from build123d import *

# Parameters (mm, degrees)
BOSS_EXTRUDE2_DEPTH      = 10
BOSS_EXTRUDE2_DEPTH_BACK = 14
SKETCH2_R                = 25
SKETCH4_R                = 62.5
BOSS_EXTRUDE3_DEPTH      = 7
BOSS_EXTRUDE3_TAPER      = 25
SKETCH6_R                = 3.5
CUT_EXTRUDE2_DEPTH       = 5


with BuildPart() as part:
    # Sketch2 → Boss-Extrude2 (new, two sides: drawn at the far end of the back side and taken through both)
    with BuildSketch(Plane.XY.offset(-BOSS_EXTRUDE2_DEPTH_BACK)):
        Circle(SKETCH2_R)
    extrude(amount=BOSS_EXTRUDE2_DEPTH + BOSS_EXTRUDE2_DEPTH_BACK)

    # Sketch4 → Boss-Extrude3 (add)
    with BuildSketch(Plane.XY.offset(10)):
        Circle(SKETCH4_R)
    extrude(amount=BOSS_EXTRUDE3_DEPTH, taper=BOSS_EXTRUDE3_TAPER)

    # Sketch6 → Cut-Extrude2 (cut)
    with BuildSketch(Plane.XY.offset(17)):
        with Locations((-50, 0)):
            Circle(SKETCH6_R)
    extrude(amount=-CUT_EXTRUDE2_DEPTH, mode=Mode.SUBTRACT)


solid = part.part
Model file for the job. Use its own axes, mm. A direction names the side the tool comes from. Coordinates: 2 decimals unless noted, no trailing zeros. Loops run counter-clockwise (first coordinate to the right, second up) from the corner with the lowest first, then second, coordinate; pieces in that order, holes last. Notation, with made-up numbers: (-4, 20.25) -> (11, 20.25) arc R13 ccw to (11, 30.25) -> close; hole circle Ø11 at (-36.5, 17). An arc over 180 degrees is marked (long way). Use one line per item in the form item = value. Start each with the question number.
(1) Cut at C-C on z = -7.5. Give the cut face in (x, y).
(2) Tool access for faces 5 (the flat face through (27, 1, 10)), 6 (the conical face through (-7.73, 58.89, 16.66)): list every direction of +Z, -Z, +X, -X, +Y, -Y with a clear straight run to the whole face (end or side of a thin tool).
(3) Probe probe 1 along Z at (x, y) = (-19, 33.5); probe 2 along Y at (x, z) = (-50, 14.95); probe 3 along Y at (x, z) = (-50, 14.4). List the from-to ranges inside material, lowest first. Write a range as from..to.
(4) Flat gauge pins, fed straight in: pin 1 (8 mm diameter, centred on x = -41, z = 11.5, fed in from +Y); pin 2 (6 mm diameter, centred on x = 18, z = -0.5, fed in from +Y); pin 3 (5.5 mm diameter, centred on x = -50, y = 0, fed in from -Z). Where does each tip first touch, or does it go through?
(5) Cut at A-A on y = 0. Give the cut face in (x, z), and give its area (3 significant figures).
(6) Pull direction X, two halves, no side cores. Call faces 1 (the cylindrical face through (23.846, 7.509, -2.168)), 2 (the flat face through (-1, 1, 17)), 3 (the cylindrical face through (-53.497, 0.154, 14.535)), 4 (the flat face through (-50, 0, 12)): pulls with the +X half, pulls with the -X half, needs draft (parallel to the pull), parting line crosses it, or undercut.
(7) Cut at B-B on x = 0. Give the cut face in (y, z), and give its area (3 significant figures).
Values:
q1.outline = circle Ø50 at (0, 0)
q2.face_5 = -Z
q2.face_6 = +Z
q3.probe_1 = 10..17
q3.probe_2 = -33.51..-3.5, 3.5..33.51
q3.probe_3 = -33.97..-3.5, 3.5..33.97
q4.pin_1 = 50.16
q4.pin_2 = 20
q4.pin_3 = 10
q5.outline = (-62.5, 10) -> (-25, 10) -> (-25, -14) -> (25, -14) -> (25, 10) -> (62.5, 10) -> (59.24, 17) -> (-46.5, 17) -> (-46.5, 12) -> (-53.5, 12) -> (-53.5, 17) -> (-59.24, 17) -> close
q5.area = 2,020 mm2
q6.face_1 = parting line crosses it
q6.face_2 = needs draft
q6.face_3 = undercut
q6.face_4 = undercut
q7.outline = (-62.5, 10) -> (-25, 10) -> (-25, -14) -> (25, -14) -> (25, 10) -> (62.5, 10) -> (59.24, 17) -> (-59.24, 17) -> close
q7.area = 2,050 mm2
